Job drawing, mm, ordinate dimensions from the low corner. One solid piece. A direction names the side the tool comes from. Give positions to 0.01 mm unless a question says otherwise; leave off trailing zeros. Loops run counter-clockwise (first coordinate to the right, second up) from the corner with the lowest first, then second, coordinate; pieces in that order, holes last. Notation, with made-up numbers: M 41,45.25 L 88,45.25 A25 cw 88,73.25 Z; hole C 87,47.25 d5. An arc over 180 degrees is marked long. Put each result on its own line as item: value.
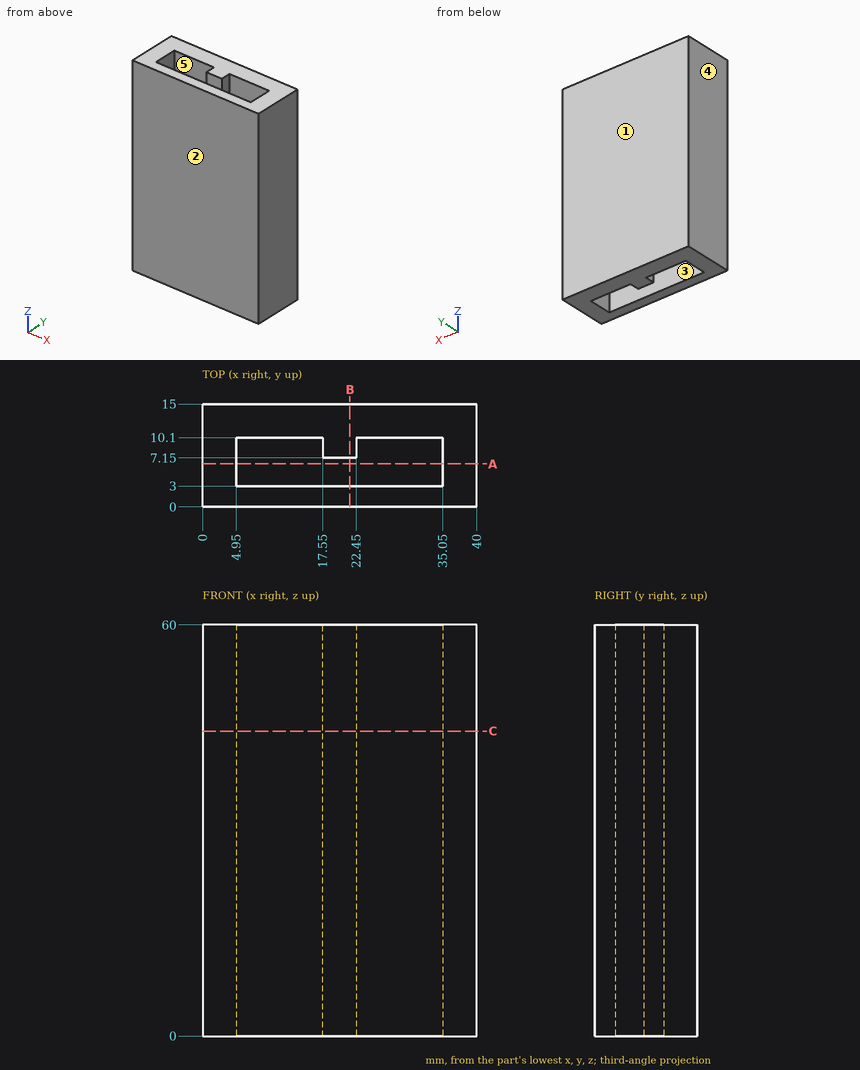
Q1. Slice it at B-B (x = 21.5). List the corners of the cut face in (y, z).
Here are the results:
outline: M 0,0 L 3,0 L 3,60 L 0,60 Z; M 7.15,0 L 15,0 L 15,60 L 7.15,60 Z
Q2. Tool access for the marked faces 4 and 5: list every direction of +Z, -Z, +X, -X, +Y, -Y with a clear straight run to the whole face (end or side of a thin tool).
Here are the results:
face 4: +Z, -Z, -X, +Y, -Y
face 5: +Z, -Z
Q3. Slice it at A-A (y = 6.25). List the corners of the cut face in (x, z).
Here are the results:
outline: M 0,0 L 4.95,0 L 4.95,60 L 0,60 Z; M 35.05,0 L 40,0 L 40,60 L 35.05,60 Z
Q4. Mould opens along Y. For the marked faces 1, 2 and 3 say: pulls with the +Y half, pulls with the -Y half, needs draft (parallel to the pull), parting line crosses it, or undercut.
Here are the results:
face 1: pulls with the +Y half
face 2: pulls with the -Y half
face 3: undercut
Q5. Slice it at C-C (z = 44.5). List the corners of the cut face in (x, y).
Here are the results:
outline: M 0,0 L 40,0 L 40,15 L 0,15 Z; hole M 4.95,3 L 35.05,3 L 35.05,10.1 L 22.45,10.1 L 22.45,7.15 L 17.55,7.15 L 17.55,10.1 L 4.95,10.1 Z
Q6. Probe line 1 (X direction, y = 8.25, z = 56); line 2 (X direction, y = 7, z = 50); line 3 (Y direction, x = 28, z = 30.5). List the from-to ranges inside material, lowest first. Write a range as from..to.
Here are the results:
line 1: 0..4.95, 17.55..22.45, 35.05..40
line 2: 0..4.95, 35.05..40
line 3: 0..3, 10.1..15
